Autodesk Inventor part; units mm, degrees
ref_plane "YZ Plane" through (0, 0, 0) normal (1, 0, 0) x (0, 1, 0)
ref_plane "XZ Plane" through (0, 0, 0) normal (0, 1, 0) x (-1, 0, 0)
ref_plane "XY Plane" through (0, 0, 0) normal (0, 0, 1) x (1, 0, 0)
sketch "Boceto1" plane through (0, 0, 0) normal (1, 0, 0) x (0, 1, 0)
  line L0 (0, 0) -> (0, 125)
  line L1 (0, 0) -> (125, 0) construction
  line L2 (0, 0) -> (0, -125)
  line L3 (0, 0) -> (125, 0) construction
  line L4 (0, 0) -> (-20, 0)
  line L5 (0, 0) -> (20, 0) construction
  line L6 (0, 0) -> (500, 0) construction
  line L7 (0, 0) -> (-20, 0)
  line L8 (0, 0) -> (20, 0) construction
  line L9 (0, 0) -> (0, -246.4363)
  line L10 (0, 0) -> (246.4363, 0) construction
  line L11 (0, 0) -> (0, 250)
  line L12 (0, 0) -> (250, 0) construction
  arc A0 (0, 250) -> (0, -246.4363) centre (1530.2267, 1.7819) ccw
  line L13 (0, 125) -> (-100, 125)
  line L14 (0, 125) -> (100, 125) construction
  line L15 (0, 250) -> (-5, 250)
  line L16 (0, 250) -> (5, 250) construction
  line L17 (0, -246.4363) -> (-5, -246.4363)
  line L18 (-20, 0) -> (-23, 0)
  line L19 (-20, 0) -> (-17, 0) construction
  line L20 (-20, 0) -> (-25, 0)
  line L21 (-20, 0) -> (-15, 0) construction
  arc A1 (-5, 250) -> (-5, -246.4363) centre (1525.2267, 1.7819) ccw
  point P0 (-20.0963, 125)
  point P1 (-15.0963, 125)
  dimension "d14" = 100
  dimension "d15" = 180
  dimension "d16" = 5
  dimension "d17" = 180
  dimension "d18" = 5
  dimension "d19" = 3
  dimension "d20" = 180
  dimension "d21" = 5
  dimension "d22" = 180
revolve "Revolución1" add sketch "Boceto1" angle 90 about axis through (0, -20, 0) along (0, -1, 0) contours L18 L20 A1 L13 A0
fillet "Empalme1" [suppressed]
sketch "Boceto2" plane through (0, -25, 0) normal (1, 0, 0) x (0, 0, -1)
  line L0 (0, -0.001) -> (0, 4.7578)
  line L1 (0, -0.001) -> (25, -0.001) construction
  line L2 (0, -0.001) -> (0, -25.001)
  line L3 (0, -0.001) -> (25, -0.001) construction
  line L4 (-25, -50.001) -> (25, -50.001)
  line L5 (25, -50.001) -> (25, -0.001)
  line L6 (-25, -0.001) -> (-25, -50.001)
  line L7 (-25, -50.001) -> (25, -0.001) construction
  line L8 (25, -50.001) -> (-25, -0.001) construction
  arc A0 (-250.0001, 20) -> (246.437, 19.9995) centre (-1.7798, 1550.1723) ccw
  line L9 (-25, -0.001) -> (-25, 0.2817)
  line L10 (25, -0.001) -> (25, 0.5411)
  line L11 (0, -50.001) -> (0, -35.001)
  line L12 (0, -50.001) -> (15, -50.001) construction
  circle A1 centre (0, -35.001) radius 6
  line L13 (0, -35.001) -> (-20, -35.001)
  line L14 (0, -35.001) -> (20, -35.001) construction
  circle A2 centre (-20, -35.001) radius 2.5
  line L15 (-20.4375, -32.5396) -> (-1.05, -29.0936)
  line L16 (-20.4375, -37.4624) -> (0, -41.0951)
  line L17 (0, -35.001) -> (0, -29.001)
  line L18 (25, -50.001) -> (-25, -0.001) construction
  circle A3 centre (0, -35.001) radius 6
  line L19 (0, -35.001) -> (20, -35.001)
  circle A4 centre (20, -35.001) radius 2.5
  line L20 (20.4375, -32.5396) -> (1.05, -29.0936)
  line L21 (20.4375, -37.4624) -> (0, -41.0951)
  point P0 (0, 25)
  point P1 (0, 0)
  point P2 (-20.2213, -32.5012)
  point P3 (20.2213, -32.5012)
  point P4 (1.05, -29.0936)
  point P5 (25, 0.2293)
  point P6 (-25, 0.1719)
  point P7 (0, 4.9037)
  point P8 (-1.05, -40.9084)
  point P9 (1.05, -40.9084)
  dimension "d25" = 25
  dimension "d27" = 25
  dimension "d28" = 90
  dimension "d29" = 50
  dimension "d30" = 50
  dimension "d31" = 15
  dimension "d32" = 90
  dimension "d33" = 12
  dimension "d34" = 20
  dimension "d35" = 180
  dimension "d36" = 5
extrude "Extrusión1" add sketch "Boceto2" along normal blind 10
extrude "Extrusión2" add sketch "Boceto2" along normal blind 6 contours A1 L13 L11 | L11 L19 A1 | L16 A2 L13 A1 | A1 L19 A4 L21 | L13 A1 L17 | L17 A1 L19 | L13 A2 L15 A1 | A1 L20 A4 L19 | A4
sketch "Boceto3" plane through (0, -25, 0) normal (1, 0, 0) x (0, 0, -1)
  arc A0 (-25, 0.1719) -> (25, 0.2293) centre (-1.7798, 1550.1723) ccw
  line L0 (0, -0.001) -> (-143.598, -0.001)
  line L1 (-143.598, -0.001) -> (-143.598, 29.4802)
  line L2 (-143.598, 29.4802) -> (0, 29.4802)
  line L3 (0, 29.4802) -> (0, -0.001)
  point P0 (0, 25)
extrude "Extrusión3" cut sketch "Boceto3" against normal blind 152
Work out the finished part from the listing and answer in its coordinate system (mm). A direction names the side the tool comes from. Round coordinates to 2 decimals unless told otherwise and drop trailing zeros. Loops run counter-clockwise (first coordinate to the right, second up) from the corner with the lowest first, then second, coordinate; pieces in that order, holes last. Notation, with made-up numbers: (31.5, 34.5) -> (51.5, 34.5) arc R31 cw to (51.5, 59.5) -> close; hole circle Ø6 at (22.5, 84.5). An arc over 180 degrees is marked (long way). Use one line per item in the form item = value.
(1) For a pull along Y with two mould halves and no side action, classify faces 3 (the cylindrical face through (5, -25, 0)), 4 (the flat face through (10, -50, 0)), 5 (the flat face through (7.152, -64.253, 10.362)) as released by +Y, released by -Y, zero draft, split by the parting line, or undercut.
Answer list:
face_3 = released by +Y
face_4 = zero draft
face_5 = undercut
(2) A flat-ended cylindrical pin translates along its axis: P1, Ø3, axis at y = -60.001, z = 20, coming from the -X side. Find the tip coordinate at first contact, or state that the pin passes through.
Answer list:
P1 = through
(3) Find section C-C on y = -65. Give the vertices of the cut face in (x, z).
Answer list:
outline = (0, -25) -> (10, -25) -> (10, -6.16) -> (6, -6.16) -> (6, 6.16) -> (10, 6.16) -> (10, 25) -> (0, 25) -> close
(4) A tool of negligible diameter and unlimited length cuts with its end or side. For faces 1 (the cylindrical face through (8, -54, 0)), 2 (the flat face through (0, -50, 0)), from which of +Z, -Z, +X, -X, +Y, -Y can it reach the whole face along a straight path? Write none if from no direction.
Answer list:
face_1 = +X
face_2 = +Z, -Z, -X, +Y, -Y
(5) Find section B-B on x = 8. Give the vertices of the cut face in (y, z).
Answer list:
outline = (-75, -25) -> (-24.77, -25) arc R1550.17 cw to (-24.83, 25) -> (-75, 25) -> close; hole (-66.1, 0) -> (-62.46, -20.44) arc R2.5 ccw to (-57.54, -20.44) -> (-54.09, -1.05) arc R6 ccw to (-54.09, 1.05) -> (-57.54, 20.44) arc R2.5 ccw to (-62.46, 20.44) -> close
(6) Straight lines are drawn through the part: line 1 (X direction, y = -65, z = -1.5); line 2 (Y direction, x = 4.25, z = 20) (3 decimals); line 3 (Y direction, x = 2.25, z = -21). For each, find the intervals that lie inside material, in ascending order.
Answer list:
line_1 = 0 to 6
line_2 = -75.001 to -62.501, -57.501 to -24.895
line_3 = -75 to -24.83
(7) Find section A-A on z = 8.5. Give the vertices of the cut face in (x, y).
Answer list:
outline = (0, -75) -> (10, -75) -> (10, -64.58) -> (6, -64.58) -> (6, -55.42) -> (10, -55.42) -> (10, -24.99) -> (0, -24.99) -> close
